from build123d import *

# Parameters (mm, degrees)
F1_DEPTH  = 16.51
F3_DEPTH  = 6.35
F4_R      = 0.635
F5_DEPTH  = 1.5691231
F6_R      = 2.53999
F7_R      = 0.635
F9_DEPTH  = 6.35
F11_D     = 2.54
F16_D     = 127
F16_DEPTH = 14.606


# Not quite as in the source:
# - a fillet or chamfer is up to 0.001 mm smaller than in the source, because OpenCascade refuses the exact size
# - a length typed as a fraction of an inch, garbled in the dataset ("3 / 203.2 mm" for 3/8 in), is restored
# - the program builds the solid bodies; features that only make, move or delete a surface that nothing else refers to are left out


with BuildPart() as f1:
    # F0 (on Top) → F1 (new body)
    with BuildSketch(Plane.XY):
        Polygon((5.5418181818, 9.525), (0, 9.525), (-5.5418181818, 9.525), (-11.6647200825, 3.4020980993), (-11.6647200825, 0), (-11.6647200825, -3.4020980993), (-5.5418181818, -9.525), (0, -9.525), (5.5418181818, -9.525), (11.6647200825, -3.4020980993), (11.6647200825, 0), (11.6647200825, 3.4020980993), align=None)
        with BuildLine():
            ThreePointArc((5.4764899478, 7.7931818182), (8.4524905132, 4.3910168667), (9.525, 0))
            ThreePointArc((9.525, 0), (8.4524905132, -4.3910168667), (5.4764899478, -7.7931818182))
            Line((5.4764899478, -7.7931818182), (0, -7.7931818182))
            Line((0, -7.7931818182), (-5.4764899478, -7.7931818182))
            ThreePointArc((-5.4764899478, -7.7931818182), (-8.4524905132, -4.3910168667), (-9.525, 0))
            ThreePointArc((-9.525, 0), (-8.4524905132, 4.3910168667), (-5.4764899478, 7.7931818182))
            Line((-5.4764899478, 7.7931818182), (0, 7.7931818182))
            Line((0, 7.7931818182), (5.4764899478, 7.7931818182))
        make_face(mode=Mode.SUBTRACT)
    extrude(amount=F1_DEPTH)

    # F2 (on Top) → F3 (join)
    with BuildSketch(Plane.XY):
        Polygon((11.0941231, -2.54), (11.0941231, 0), (11.0941231, 2.54), (9.525, 2.54), (9.525, 0), (9.525, -2.54), align=None)
    extrude(amount=-F3_DEPTH)

    # F4 (on face) → F5 (join)
    with BuildSketch(Plane.YZ.offset(11.0941231)):
        with Locations((0, -5.08)):
            Circle(F4_R)
    extrude(amount=F5_DEPTH)

    # F6 (radius 2.54 in the source; OpenCascade refuses exactly that, so slightly less here)
    f6_edges = [f1.edges().sort_by_distance(p)[0] for p in [
        (10.309562, -2.54, -6.35),
        (10.309562, 2.54, -6.35),
    ]]
    fillet(f6_edges, radius=F6_R)

    # F7
    f7_edges = [f1.edges().sort_by_distance(p)[0] for p in [
        (12.663246, -0.635, -5.08),
    ]]
    fillet(f7_edges, radius=F7_R)

    # F8 (on face) → F9 (join)
    with BuildSketch(Plane.XY.offset(16.51)):
        Polygon((11.6647200825, 2.54), (10.095592022, 2.54), (10.095592022, 0), (10.095592022, -2.54), (11.6647200825, -2.54), (11.6647200825, 0), align=None)
    extrude(amount=F9_DEPTH)

    # F11 (through all)
    with Locations(Plane.YZ.offset(11.6647200825)):
        with Locations((0, 20.32)):
            Hole(F11_D / 2)

    # F12: F1 across plane


with BuildPart() as f1_1:
    add(f1.part)
    add(f1.part.mirror(Plane.YZ))

    # F16 (through all, one way)
    with BuildSketch(Plane(origin=(0, 0, 8.255), x_dir=(1, 0, 0), z_dir=(0, 0, -1))):
        with Locations((0, 0)):
            Circle(F16_D / 2)
    extrude(amount=-F16_DEPTH, mode=Mode.SUBTRACT)


solid = f1_1.part
Build history of the part. All positions in model axes, mm. A direction names the side the tool comes from. Give positions to 0.01 mm unless a question says otherwise; leave off trailing zeros. Order: outer loops, then holes, each group sorted by start corner. A loop starts at its lowest first (then second) coordinate and runs counter-clockwise, first axis right, second up. Notation, with made-up numbers: M 21.5,6.25 L 75.5,6.25 A31 cw 75.5,31.25 Z; hole C 68.25,-30 d5. An arc over 180 degrees is marked long. Use one line per item in the form item = value.
1) Saw through at C-C (z = 4.25). Give the cut face in (x, y) (3 decimals).
Calculated:
outline = M -11.665,-3.402 L -5.542,-9.525 L 5.542,-9.525 L 11.665,-3.402 L 11.665,3.402 L 5.542,9.525 L -5.542,9.525 L -11.665,3.402 Z; hole M -5.476,-7.793 L 5.476,-7.793 A9.525 ccw 5.476,7.793 L -5.476,7.793 A9.525 ccw Z
2) Saw through at D-D (z = -5.08). Give the cut face in (x, y) (3 decimals).
Calculated:
outline = M -12.028,-0.635 L -11.094,-0.635 L -11.094,-2.2 L -9.525,-2.2 L -9.525,2.2 L -11.094,2.2 L -11.094,0.635 L -12.028,0.635 A0.635 ccw Z; M 9.525,-2.2 L 11.094,-2.2 L 11.094,-0.635 L 12.028,-0.635 A0.635 ccw 12.028,0.635 L 11.094,0.635 L 11.094,2.2 L 9.525,2.2 Z
3) Saw through at A-A (x = 3). Give the cut face in (y, z) (3 decimals).
Calculated:
outline = M -9.525,0 L -7.793,0 L -7.793,8.255 L -9.525,8.255 Z; M 7.793,0 L 9.525,0 L 9.525,8.255 L 7.793,8.255 Z
4) Drop flat-ended pins along their axis: pin 1 (2 mm diameter, centred on y = 7, z = 3.5, fed in from +X); pin 2 (3 mm diameter, centred on y = -3, z = 0.5, fed in from -X); pin 3 (5 mm diameter, centred on x = -4.5, y = -7, fed in from -Z). Give the stop position or say it passes through.
Calculated:
pin_1 = 9.07
pin_2 = -11.66
pin_3 = 0
5) Tool access for faces 1 (the face through (0, -7.793, 4)), 2 (the face through (-10, -2.54, -2)), 3 (the face through (10, 2.54, -2)), 4 (the face through (9.525, 0, -3)): list every direction of +Z, -Z, +X, -X, +Y, -Y with a clear straight run to the whole face (end or side of a thin tool).
Calculated:
face_1 = +Z, -Z
face_2 = -Z, +X, -X, -Y
face_3 = -Z, +X, -X, +Y
face_4 = -Z, +Y, -Y
6) Probe probe 1 along Y at (x, z) = (3, 7) (3 decimals); probe 2 along X at (y, z) = (0, -1) (3 decimals); probe 3 along Z at (x, y) = (-8.5, -6) (3 decimals). List the from-to ranges inside material, lowest first.
Calculated:
probe_1 = -9.525 to -7.793, 7.793 to 9.525
probe_2 = -11.094 to -9.525, 9.525 to 11.094
probe_3 = 0 to 8.255
7) Saw through at B-B (y = 5.25). Give the cut face in (x, z) (3 decimals), plus the area to 3 significant figures.
Calculated:
outline = M -9.817,0 L -7.948,0 L -7.948,8.255 L -9.817,8.255 Z; M 7.948,0 L 9.817,0 L 9.817,8.255 L 7.948,8.255 Z
area = 30.9 mm2
8) Two-plate mould, pull along X, no slides. Class faces 5 (the face through (-11.094, 0, -3)), 6 (the face through (-10, 2.54, -2)), 7 (the face through (0, 7.793, 4)): released by +X, released by -X, zero draft, split by the parting line, or undercut.
Calculated:
face_5 = released by -X
face_6 = zero draft
face_7 = undercut
